from build123d import *

# Parameters (mm, degrees)
MAIN_BLOCK_DEPTH                 = 5
BELT_START                       = -1
BELT_CLAMP_CUTOUT_SKETCH_W       = 15
BELT_CLAMP_CUTOUT_SKETCH_H       = 6.3
BELT_CLAMP_CUTOUT_DEPTH          = 1
BELT_CLAMP_SCREW_HOLES_D         = 3.2
BELT_CLAMP_SCREW_NUT_TRAPS_DEPTH = 2.3
BELT_GUIDE_CHAMFERS_SIZE         = 1
RAIL_MOUNT_BLOCK_SKETCH_W        = 45.4
RAIL_MOUNT_BLOCK_SKETCH_H        = 5
CARRIAGE_MOUNTING_BLOCK_DEPTH    = 27
CARRIAGE_MOUNTING_HOLES_D        = 3.2


with BuildPart() as part:
    # Main Block Sketch → Main Block (new body)
    with BuildSketch(Plane(origin=(30.899718474, 0, 0), x_dir=(0, 0, -1), z_dir=(1, 0, 0))):
        Polygon((-55.037241551, 38.898583536), (-9.637241551, 38.898583536), (-9.637241551, 33.898583536), (-9.637241551, 0.898583536), (-55.037241551, 0.898583536), (-55.037241551, 33.898583536), align=None)
    extrude(amount=MAIN_BLOCK_DEPTH)

    # Belt Clamp Cutout Sketch → Belt Clamp Cutout (cut)
    with BuildSketch(Plane(origin=(35.899718474, 0, 0), x_dir=(0, 0, -1), z_dir=(1, 0, 0)).offset(BELT_START)):
        with Locations((-47.537241551, 7.898583536)):
            Rectangle(BELT_CLAMP_CUTOUT_SKETCH_W, BELT_CLAMP_CUTOUT_SKETCH_H)
        with Locations((-17.137241551, 7.898583536)):
            Rectangle(BELT_CLAMP_CUTOUT_SKETCH_W, BELT_CLAMP_CUTOUT_SKETCH_H)
        with Locations((-17.137241551, 18.198583536)):
            Rectangle(BELT_CLAMP_CUTOUT_SKETCH_W, BELT_CLAMP_CUTOUT_SKETCH_H)
        with Locations((-47.537241551, 18.198583536)):
            Rectangle(BELT_CLAMP_CUTOUT_SKETCH_W, BELT_CLAMP_CUTOUT_SKETCH_H)
    extrude(amount=BELT_CLAMP_CUTOUT_DEPTH, mode=Mode.SUBTRACT)

    # Belt Clamp Screw Holes (through all)
    with Locations(Plane(origin=(35.899718474, 0, 0), x_dir=(0, 0, -1), z_dir=(1, 0, 0))):
        with Locations((-47.537241551, 13.048583536), (-17.137241551, 13.048583536), (-32.337241551, 13.048583536)):
            Hole(BELT_CLAMP_SCREW_HOLES_D / 2)

    # Nut Trap Sketch → Belt Clamp Screw Nut Traps (cut)
    with BuildSketch(Plane(origin=(30.899718474, 0, 0), x_dir=(0, 0, -1), z_dir=(1, 0, 0))):
        Polygon((-45.978395824, 15.748583536), (-49.096087278, 15.748583536), (-50.654933005, 13.048583536), (-49.096087278, 10.348583536), (-45.978395824, 10.348583536), (-44.419550097, 13.048583536), align=None)
        Polygon((-30.778395824, 15.748583536), (-33.896087278, 15.748583536), (-35.454933005, 13.048583536), (-33.896087278, 10.348583536), (-30.778395824, 10.348583536), (-29.219550097, 13.048583536), align=None)
        Polygon((-15.578395824, 15.748583536), (-18.696087278, 15.748583536), (-20.254933005, 13.048583536), (-18.696087278, 10.348583536), (-15.578395824, 10.348583536), (-14.019550097, 13.048583536), align=None)
    extrude(amount=BELT_CLAMP_SCREW_NUT_TRAPS_DEPTH, mode=Mode.SUBTRACT)

    # Belt Guide Chamfers
    belt_guide_chamfers_edges = [part.edges().sort_by_distance(p)[0] for p in [
        (34.899718474, 7.898583536, 40.037241551),
        (34.899718474, 18.198583536, 40.037241551),
        (34.899718474, 7.898583536, 24.637241551),
        (34.899718474, 18.198583536, 24.637241551),
    ]]
    chamfer(belt_guide_chamfers_edges, length=BELT_GUIDE_CHAMFERS_SIZE - 0.0001)  # a hair under: the kernel refuses the full size
    belt_guide_chamfers_2_edges = [part.edges().sort_by_distance(p)[0] for p in [
        (34.899718474, 18.198583536, 55.037241551),
        (34.899718474, 7.898583536, 55.037241551),
        (34.899718474, 7.898583536, 9.637241551),
        (34.899718474, 18.198583536, 9.637241551),
    ]]
    chamfer(belt_guide_chamfers_2_edges, length=BELT_GUIDE_CHAMFERS_SIZE)

    # Rail Mount Block Sketch → Carriage Mounting Block (add)
    with BuildSketch(Plane(origin=(30.899718474, 0, 0), x_dir=(0, 0, -1), z_dir=(1, 0, 0))):
        with Locations((-32.337241551, 36.398583536)):
            Rectangle(RAIL_MOUNT_BLOCK_SKETCH_W, RAIL_MOUNT_BLOCK_SKETCH_H)
    extrude(amount=-CARRIAGE_MOUNTING_BLOCK_DEPTH)

    # Carriage Mounting Holes (through all)
    with Locations(Plane(origin=(0, 38.898583536, 0), x_dir=(1, 0, 0), z_dir=(0, 1, 0))):
        with Locations((7.399718474, -42.337241551), (27.399718474, -42.337241551), (7.399718474, -22.337241551), (27.399718474, -22.337241551)):
            Hole(CARRIAGE_MOUNTING_HOLES_D / 2)


solid = part.part
Check sheet for the modelled part. Datum: model origin and axes. Units: mm. A direction names the side the tool comes from. Round coordinates to 2 decimals unless told otherwise and drop trailing zeros. Loops run counter-clockwise (first coordinate to the right, second up) from the corner with the lowest first, then second, coordinate; pieces in that order, holes last.
1. Mould release check, pull along Y, two halves, no side actions. Record for faces 6 (the flat face through (32, 11.7, 14.8)), 7 (the flat face through (35.9, 20, 32)): released by +Y, released by -Y, zero draft, split by the parting line, or undercut.
2. Sectioned sample at D-D on z = 38. Record the boundary of the cut face in (x, y).
3. Gauge pin test, flat ends, axial feed: pin 1 Ø6 at (y, z) = (7, 43.5) entering from +X; pin 2 Ø4 at (y, z) = (13.05, 47.54) entering from -X; pin 3 Ø3 at (y, z) = (19.5, 18) entering from +X; pin 4 Ø4 at (x, z) = (24.5, 50.5) entering from -Y. Record the tip position at first contact, or that the pin passes through.
4. Sectioned sample at A-A on x = 6.5. Record the boundary of the cut face in (y, z).
5. Scan lines: probe 1 along Y at (x, z) = (31, 17); probe 2 along Z at (x, y) = (8.5, 35); probe 3 along X at (y, z) = (19, 47.5). Record each from-to range of solid material in increasing order.
6. Sectioned sample at B-B on z = 47.5. Record the boundary of the cut face in (x, y), and give its area (3 significant figures).
7. Set-up check for faces 1 (the flat face through (35.3, 11.049, 47.6)), 2 (the flat face through (35.3, 4.749, 17.2)), 3 (the flat face through (32, 28, 9.637)), 4 (the flat face through (32, 10.349, 32)), 5 (the cylindrical face through (34.53, 11.63, 17.88)): record each of +Z, -Z, +X, -X, +Y, -Y from which the full face is reachable in a straight line by a thin tool's end or side.
8. Sectioned sample at C-C on y = 12.5. Record the boundary of the cut face in (x, z).
Recorded:
1. face 6: undercut
1. face 7: zero draft
2. outline: (3.9, 33.9) - (30.9, 33.9) - (30.9, 0.9) - (35.9, 0.9) - (35.9, 38.9) - (3.9, 38.9) - close
3. pin 1: stops at x = 35.9
3. pin 2: stops at x = 33.2
3. pin 3: stops at x = 34.9
3. pin 4: stops at y = 33.9
4. outline: (33.9, 9.64) - (38.9, 9.64) - (38.9, 21.01) - (33.9, 21.01) - close; (33.9, 23.66) - (38.9, 23.66) - (38.9, 41.01) - (33.9, 41.01) - close; (33.9, 43.66) - (38.9, 43.66) - (38.9, 55.04) - (33.9, 55.04) - close
5. probe 1: y = 0.9 to 10.35, 15.75 to 38.9
5. probe 2: z = 9.64 to 21.18, 23.5 to 41.18, 43.5 to 55.04
5. probe 3: x = 30.9 to 34.9
6. outline: (3.9, 33.9) - (30.9, 33.9) - (30.9, 15.75) - (33.2, 15.75) - (33.2, 14.65) - (35.9, 14.65) - (35.9, 15.05) - (34.9, 15.05) - (34.9, 21.35) - (35.9, 21.35) - (35.9, 38.9) - (3.9, 38.9) - close; (30.9, 0.9) - (35.9, 0.9) - (35.9, 4.75) - (34.9, 4.75) - (34.9, 11.05) - (35.9, 11.05) - (35.9, 11.45) - (33.2, 11.45) - (33.2, 10.35) - (30.9, 10.35) - close
6. area: 291 mm2
7. face 1: +Z, +X
7. face 2: -Z, +X
7. face 3: -Z, +X, -X, +Y, -Y
7. face 4: -X
7. face 5: +X, -X
8. outline: (30.9, 9.64) - (35.9, 9.64) - (35.9, 15.63) - (33.2, 15.63) - (33.2, 14.34) - (30.9, 14.34) - close; (30.9, 19.94) - (33.2, 19.94) - (33.2, 18.64) - (35.9, 18.64) - (35.9, 30.83) - (33.2, 30.83) - (33.2, 29.54) - (30.9, 29.54) - close; (30.9, 35.14) - (33.2, 35.14) - (33.2, 33.84) - (35.9, 33.84) - (35.9, 46.03) - (33.2, 46.03) - (33.2, 44.74) - (30.9, 44.74) - close; (30.9, 50.34) - (33.2, 50.34) - (33.2, 49.04) - (35.9, 49.04) - (35.9, 55.04) - (30.9, 55.04) - close
